Can you work these out from the model? Positions are in its coordinate system, mm. Give positions to 0.01 mm unless a question says otherwise; leave off trailing zeros. Order: outer loops, then holes, each group sorted by start corner. A loop starts at its lowest first (then second) coordinate and runs counter-clockwise, first axis right, second up. Notation, with made-up numbers: (19.5, -15.75) - (39.5, -15.75) arc R34 ccw to (39.5, 14.25) - close; hole circle Ø3 at (8.5, 51). An arc over 180 degrees is marked (long way). Use one line per item in the form item = value. Start each with the question number.
1) Please list where these lines run through material, in increasing order: probe 1 along Y at (x, z) = (-10.5, -24); probe 2 along Z at (x, y) = (-1, 303.5); probe 3 along Y at (x, z) = (-36, -24.5).
2) Suppose I cut it at A-A, the plane z = 0. Write out the boundary of the cut face in (x, y), and give its area (3 significant figures).
3) Suppose I cut it at D-D, the plane z = 39. Write out the boundary of the cut face in (x, y), and give its area (3 significant figures).
4) For pin 1 (7.5 mm diameter, centred on x = 1, y = 382.5, fed in from +Z); pin 2 (4 mm diameter, centred on x = 7.5, z = 15, fed in from -Y); pin 3 (3 mm diameter, centred on x = 36, z = 35, fed in from +Y); pin 4 (10 mm diameter, centred on x = -0.5, y = 299.5, fed in from -Z), each with a flat end and sliding along its axis, tell me the tip position at first contact or that it passes through.
5) Suppose I cut it at B-B, the plane x = 0. Write out the boundary of the cut face in (y, z), and give its area (3 significant figures).
6) Suppose I cut it at C-C, the plane y = 627. Write out the boundary of the cut face in (x, z).
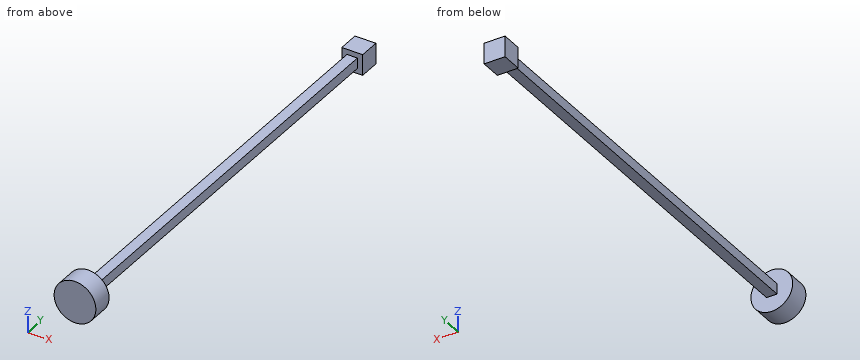
```python
from build123d import *

# Parameters (mm, degrees)
SKETCH1_R           = 50
BOSS_EXTRUDE1_DEPTH = 50
SKETCH2_W           = 25
SKETCH2_H           = 25
BOSS_EXTRUDE2_DEPTH = 1000
SKETCH3_W           = 50
SKETCH3_H           = 50
BOSS_EXTRUDE3_DEPTH = 50


with BuildPart() as part:
    # Sketch1 → Boss-Extrude1 (new body)
    with BuildSketch(Plane(origin=(0, 0, 0), x_dir=(1, 0, 0), z_dir=(0, 1, 0))):
        with Locations(Location((0, 0, 0), (0, 0, 270))):
            Circle(SKETCH1_R)
    extrude(amount=BOSS_EXTRUDE1_DEPTH)

    # Sketch2 → Boss-Extrude2 (add)
    with BuildSketch(Plane(origin=(0, 50, 0), x_dir=(1, 0, 0), z_dir=(0, 1, 0))):
        Rectangle(SKETCH2_W, SKETCH2_H)
    extrude(amount=BOSS_EXTRUDE2_DEPTH)

    # Sketch3 → Boss-Extrude3 (add)
    with BuildSketch(Plane(origin=(0, 1050, 0), x_dir=(1, 0, 0), z_dir=(0, 1, 0))):
        Rectangle(SKETCH3_W, SKETCH3_H)
    extrude(amount=BOSS_EXTRUDE3_DEPTH)


solid = part.part
```
Result sheet:
q1.probe_1 = 0 to 50, 1050 to 1100
q1.probe_2 = -12.5 to 12.5
q1.probe_3 = 0 to 50
q2.outline = (-50, 0) - (50, 0) - (50, 50) - (12.5, 50) - (12.5, 1050) - (25, 1050) - (25, 1100) - (-25, 1100) - (-25, 1050) - (-12.5, 1050) - (-12.5, 50) - (-50, 50) - close
q2.area = 32,500 mm²
q3.outline = (-31.29, 0) - (31.29, 0) - (31.29, 50) - (-31.29, 50) - close
q3.area = 3,130 mm²
q4.pin_1 = 12.5
q4.pin_2 = 0
q4.pin_3 = 50
q4.pin_4 = -12.5
q5.outline = (0, -50) - (50, -50) - (50, -12.5) - (1050, -12.5) - (1050, -25) - (1100, -25) - (1100, 25) - (1050, 25) - (1050, 12.5) - (50, 12.5) - (50, 50) - (0, 50) - close
q5.area = 32,500 mm²
q6.outline = (-12.5, -12.5) - (12.5, -12.5) - (12.5, 12.5) - (-12.5, 12.5) - close
